Could you check a few things on this drawing? It's one solid part, dimensions in mm from its lowest x, y, z. Give positions to 0.01 mm unless a question says otherwise; leave off trailing zeros. Order: outer loops, then holes, each group sorted by start corner. A loop starts at its lowest first (then second) coordinate and runs counter-clockwise, first axis right, second up. Notation, with made-up numbers: M -8,-37.75 L 28,-37.75 A16 cw 28,-30.75 Z; hole C 48.25,1.25 d9. An arc over 180 degrees is marked long. Return JSON: item names as keys, results as strings. Group by question number.
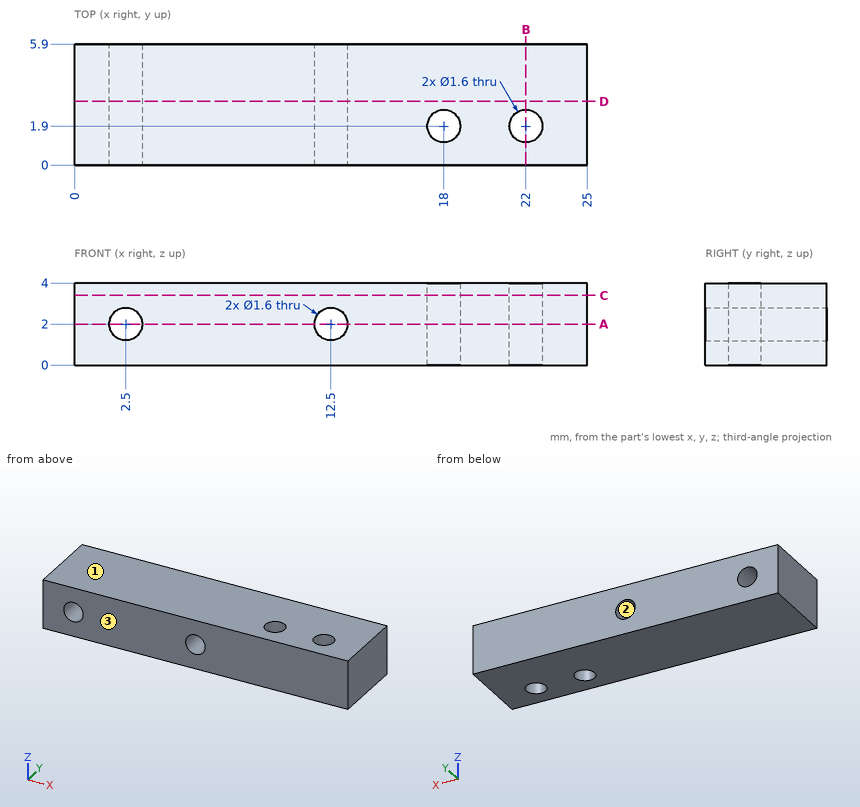
1. If we mould it in two halves opening along Z, with no side actions, what happens to the marked faces 1, 2 and 3? For each: pulls with the +Z half, pulls with the -Z half, needs draft (parallel to the pull), parting line crosses it, or undercut.
2. Imagine slicing it at B-B, the plane x = 22. Please give me the cut outline in (y, z), plus the area to 3 significant figures.
3. I need wall thicknesses on L1, parallel to X at y = 4.3, z = 2; L2, parallel to Z at x = 2.5, y = 4.15; L3, parallel to X at y = 1.95, z = 0.75. Which ranges of each line are inside material? Lowest first, please. Write a range as from..to.
4. Imagine slicing it at C-C, the plane z = 3.4. Please give me the cut outline in (x, y).
5. Imagine slicing it at D-D, the plane y = 3.1. Please give me the cut outline in (x, z).
6. Imagine slicing it at A-A, the plane z = 2. Please give me the cut outline in (x, y).
Values:
{
 "1": {"face 1": "pulls with the +Z half", "face 2": "undercut", "face 3": "needs draft"},
 "2": {"outline": "M 0,0 L 1.1,0 L 1.1,4 L 0,4 Z; M 2.7,0 L 5.9,0 L 5.9,4 L 2.7,4 Z", "area": "17.2 mm²"},
 "3": {"L1": "x = 0..1.7, 3.3..11.7, 13.3..25", "L2": "z = 0..1.2, 2.8..4", "L3": "x = 0..17.2, 18.8..21.2, 22.8..25"},
 "4": {"outline": "M 0,0 L 25,0 L 25,5.9 L 0,5.9 Z; hole C 18,1.9 d1.6; hole C 22,1.9 d1.6"},
 "5": {"outline": "M 0,0 L 25,0 L 25,4 L 0,4 Z; hole C 2.5,2 d1.6; hole C 12.5,2 d1.6"},
 "6": {"outline": "M 0,0 L 1.7,0 L 1.7,5.9 L 0,5.9 Z; M 3.3,0 L 11.7,0 L 11.7,5.9 L 3.3,5.9 Z; M 13.3,0 L 25,0 L 25,5.9 L 13.3,5.9 Z; hole C 18,1.9 d1.6; hole C 22,1.9 d1.6"}
}
